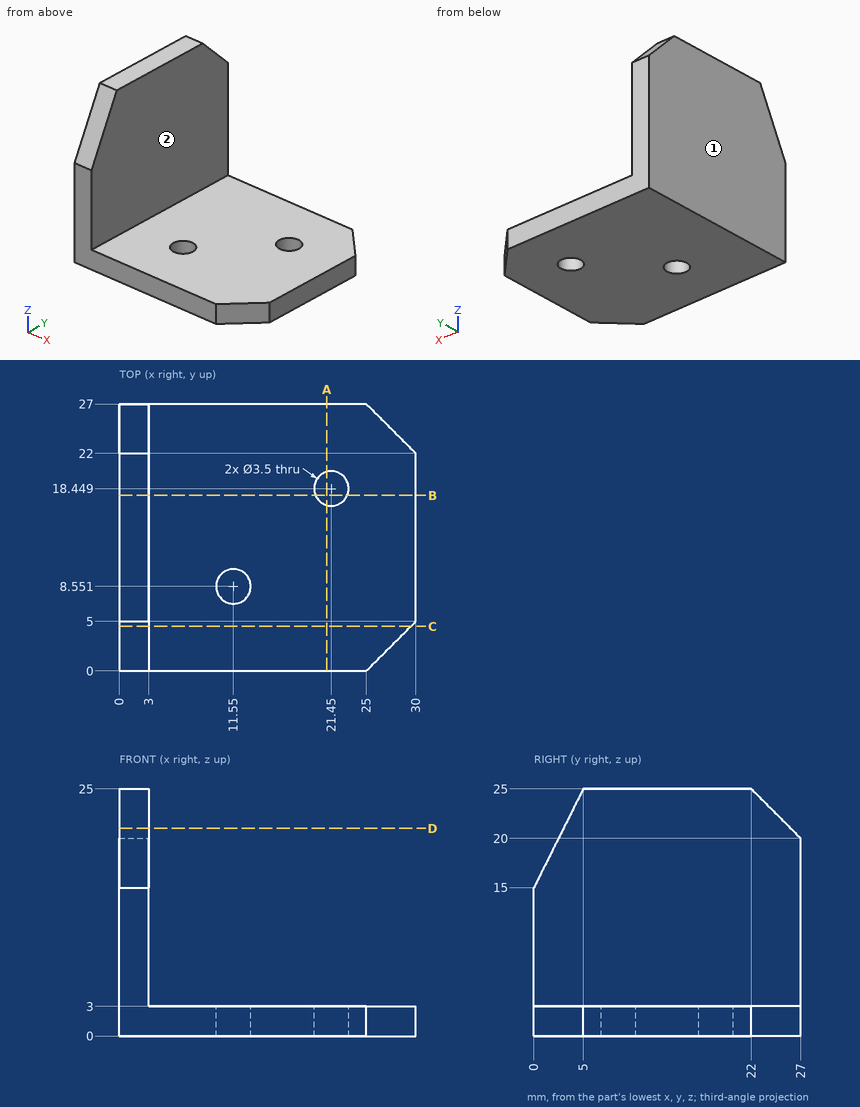
Study the drawing (mm; zero at the part's minimum x, y, z) and answer. A direction names the side the tool comes from. Give positions to 0.01 mm unless a question says otherwise; leave off trailing zeros. Loops run counter-clockwise (first coordinate to the right, second up) from the corner with the lowest first, then second, coordinate; pieces in that order, holes last. Notation, with made-up numbers: (-13.5, 75.25) - (2.5, 75.25) arc R24 ccw to (2.5, 93.25) - close; hole circle Ø2 at (-36.75, 75.5). An arc over 180 degrees is marked (long way). Answer as CSV lines item,"result". Start each with the question number.
1) Find section A-A (x = 21). Write down the section's boundary in (y, z).
2) Straight lines are drawn through the part: L1, parallel to Y at x = 21.45, z = 2.3; L2, parallel to Y at x = 11.55, z = 2.1; L3, parallel to Z at x = 26.25, y = 12.75. For each, find the intervals that lie inside material, in ascending order. Write a range as from..to.
3) Which of the six approach directions +Z, -Z, +X, -X, +Y, -Y give full straight-line access (tool end or side, diameter ignored) to the marked faces 1 and 2?
4) Find section C-C (y = 4.5). Write down the section's boundary in (x, z).
5) Each of these flat-tipped pins is pushed along its axis until it touches: pin 1 Ø6 at (x, y) = (7, 8) entering from +Z; pin 2 Ø2 at (y, z) = (10.5, 10.5) entering from +X. Where does it stop, or does it pass through?
6) Find section B-B (y = 17.75). Write down the section's boundary in (x, z) (1 decimal), then the cut area to 3 significant figures.
7) Find section D-D (z = 21). Write down the section's boundary in (x, y).
Findings below:
1,outline,"(0, 0) - (16.76, 0) - (16.76, 3) - (0, 3) - close; (20.14, 0) - (27, 0) - (27, 3) - (20.14, 3) - close"
2,L1,"0..16.7, 20.2..27"
2,L2,"0..6.8, 10.3..27"
2,L3,"0..3"
3,face 1,"+Z, -Z, -X, +Y, -Y"
3,face 2,"+Z, +X, +Y, -Y"
4,outline,"(0, 0) - (29.5, 0) - (29.5, 3) - (3, 3) - (3, 24) - (0, 24) - close"
5,pin 1,"z = 3"
5,pin 2,"x = 3"
6,outline,"(0, 0) - (19.8, 0) - (19.8, 3) - (3, 3) - (3, 25) - (0, 25) - close; (23.1, 0) - (30, 0) - (30, 3) - (23.1, 3) - close"
6,area,"146 mm^2"
7,outline,"(0, 3) - (3, 3) - (3, 26) - (0, 26) - close"
